Here's how the part is built. I have some questions about the finished solid (model axes, mm). Give positions to 0.01 mm unless a question says otherwise; leave off trailing zeros. Write each loop counter-clockwise with the first axis right and the second up, starting at its lowest first coordinate (ties: lowest second). Pieces come first, ordered by that corner, then holes. Notation, with made-up numbers: (60, 58) - (66, 58) arc R21 cw to (66, 71) - close; hole circle Ø7 at (64, -0.75). An arc over 180 degrees is marked (long way). Use a Markdown table: item, result.
Autodesk Inventor part; units mm, degrees
ref_plane "YZ Plane" through (0, 0, 0) normal (1, 0, 0) x (0, 1, 0)
ref_plane "XZ Plane" through (0, 0, 0) normal (0, 1, 0) x (-1, 0, 0)
ref_plane "XY Plane" through (0, 0, 0) normal (0, 0, 1) x (1, 0, 0)
sketch "Sketch1" plane through (0, 0, 0) normal (1, 0, 0) x (0, 1, 0)
  line L0 (0, 0) -> (380, 0)
  line L1 (400, -20) -> (400, -770)
  line L2 (380, -790) -> (0, -790)
  line L3 (0, -790) -> (0, 0)
  arc A0 (400, -20) -> (380, 0) centre (380, -20) ccw
  arc A1 (380, -790) -> (400, -770) centre (380, -770) ccw
  circle A2 centre (125, -680) radius 37.5
  line L4 (0, -170) -> (110, -170)
  line L5 (110, -270) -> (0, -270)
  line L6 (0, -270) -> (0, -170)
  arc A3 (110, -270) -> (110, -170) centre (110, -220) ccw
  line L7 (350, -680.5) -> (284.5, -680.5)
  line L8 (284.5, -680.5) -> (284.5, -650)
  line L9 (284.5, -650) -> (350, -650)
  line L10 (350, -650) -> (350, -680.5)
  line L11 (20, -588.3581) -> (20, -488.3581) construction
  line L12 (10, -588.3581) -> (10, -488.3581)
  line L13 (30, -488.3581) -> (30, -588.3581)
  arc A4 (10, -588.3581) -> (30, -588.3581) centre (20, -588.3581) ccw
  arc A5 (30, -488.3581) -> (10, -488.3581) centre (20, -488.3581) ccw
  arc A6 (10, -138.3581) -> (30, -138.3581) centre (20, -138.3581) ccw
  line L14 (20, -138.3581) -> (20, -38.3581) construction
  line L15 (10, -138.3581) -> (10, -38.3581)
  arc A7 (30, -38.3581) -> (10, -38.3581) centre (20, -38.3581) ccw
  line L16 (30, -38.3581) -> (30, -138.3581)
  point P0 (400, -790)
  point P1 (400, 0)
  point P2 (190, 0)
  point P3 (0, -270)
  point P4 (20, -538.3581)
  point P5 (30, -538.3581)
  point P6 (30, -88.3581)
  point P7 (20, -88.3581)
  dimension "d0" = 400
  dimension "d1" = 790
  dimension "d2" = 20
  dimension "d3" = 75
  dimension "d4" = 110
  dimension "d5" = 125
  dimension "d6" = 110
  dimension "d7" = 100
  dimension "d9" = 220
  dimension "d10" = 65.5
  dimension "d11" = 30.5
  dimension "d12" = 50
  dimension "d13" = 650
  dimension "d16" = 30
  dimension "d17" = 10
  dimension "d18" = 100
  dimension "d21" = 450
extrude "Extrusion1" add sketch "Sketch1" along normal blind 5 contours L0 A0 L1 A1 L2 L3 L5 A3 L4
properties part number "r2wall"
Item 1: If we section it at C-C, the plane x = 2.1: Write out the boundary of the cut face in (y, z).
Values:
| item | result |
|---|---|
| outline | (0, -790) - (380, -790) arc R20 ccw to (400, -770) - (400, -20) arc R20 ccw to (380, 0) - (0, 0) - (0, -170) - (110, -170) arc R50 cw to (110, -270) - (0, -270) - close; hole (10, -588.36) arc R10 ccw to (30, -588.36) - (30, -488.36) arc R10 ccw to (10, -488.36) - close; hole (10, -138.36) arc R10 ccw to (30, -138.36) - (30, -38.36) arc R10 ccw to (10, -38.36) - close; hole circle Ø75 at (125, -680); hole (284.5, -680.5) - (350, -680.5) - (350, -650) - (284.5, -650) - close |
Item 2: Thinking about a two-plate mould opening in Y: for faces 1 (the flat face through (0, 197, -389)), 2 (the cylindrical face through (2.46, 120.12, -717.18)), 3 (the cylindrical face through (2.465, 159.988, -218.901)), which applies, +Y half, -Y half, draft (parallel to the pull), parting line (faces both ways), or undercut?
Values:
| item | result |
|---|---|
| face 1 | draft |
| face 2 | undercut |
| face 3 | -Y half |
Item 3: If we section it at B-B, the plane y = 20: Write out the boundary of the cut face in (x, z).
Values:
| item | result |
|---|---|
| outline | (0, -790) - (5, -790) - (5, -598.36) - (0, -598.36) - close; (0, -478.36) - (5, -478.36) - (5, -270) - (0, -270) - close; (0, -170) - (5, -170) - (5, -148.36) - (0, -148.36) - close; (0, -28.36) - (5, -28.36) - (5, 0) - (0, 0) - close |
Item 4: If we section it at D-D, the plane y = 300.5: Write out the boundary of the cut face in (x, z), plus the area to 3 significant figures.
Values:
| item | result |
|---|---|
| outline | (0, -790) - (5, -790) - (5, -680.5) - (0, -680.5) - close; (0, -650) - (5, -650) - (5, 0) - (0, 0) - close |
| area | 3,800 mm2 |
Item 5: I need wall thicknesses on line 1 along Z through (x, y) = (2.1, 125); line 2 along Y through (x, z) = (3.2, -492); line 3 along Z through (x, y) = (1.05, 42.5). Which ranges of each line are inside material? Lowest first, please. Write a range as [from, to].
Values:
| item | result |
|---|---|
| line 1 | z = [-790, -717.5], [-642.5, -267.7], [-172.3, 0] |
| line 2 | y = [0, 10], [30, 400] |
| line 3 | z = [-790, -270], [-170, 0] |
Item 6: If we section it at A-A, the plane z = -63: Write out the boundary of the cut face in (x, y), plus the area to 3 significant figures.
Values:
| item | result |
|---|---|
| outline | (0, 0) - (5, 0) - (5, 10) - (0, 10) - close; (0, 30) - (5, 30) - (5, 400) - (0, 400) - close |
| area | 1,900 mm2 |
